The model under review builds one solid part; all positions refer to its coordinate system, in mm. Face numbers are marked on the shaded views. Round coordinates to 2 decimals unless told otherwise and drop trailing zeros. Write each loop counter-clockwise with the first axis right and the second up, starting at its lowest first coordinate (ties: lowest second). Pieces come first, ordered by that corner, then holes. Notation, with made-up numbers: (-26, 19.5) - (11, 19.5) arc R16 cw to (11, 39.5) - close; hole circle Ø6 at (73.5, -32.75). An arc over 180 degrees is marked (long way). Write each question's results on one line, items separated by ' | '.
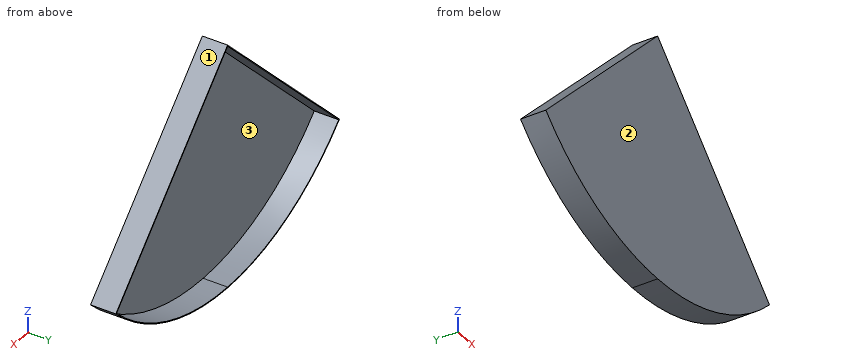
Autodesk Inventor part; units mm, degrees
ref_plane "YZ Plane" through (0, 0, 0) normal (1, 0, 0) x (0, 1, 0)
ref_plane "XZ Plane" through (0, 0, 0) normal (0, 1, 0) x (-1, 0, 0)
ref_plane "XY Plane" through (0, 0, 0) normal (0, 0, 1) x (1, 0, 0)
sketch "草圖1" plane through (0, 0, 0) normal (0, 1, 0) x (-1, 0, 0)
  line L0 (0, 0) -> (-1060.6602, -1060.6602)
  arc A0 (-1060.6602, -1060.6602) -> (0, -1500) centre (0, 0) ccw
  line L1 (0, -1935.3977) -> (0, 330.8159)
  arc A1 (-1067.7254, -1060.6543) -> (0, -1505) centre (0, 0) ccw
  line L2 (-1067.7254, -1060.6543) -> (0, 7.0711)
  line L3 (0, 0) -> (1060.6602, -1060.6602)
  arc A2 (0, -1500) -> (1060.6602, -1060.6602) centre (0, 0) ccw
  arc A3 (0, -1505) -> (1067.7254, -1060.6543) centre (0, 0) ccw
  line L4 (1067.7254, -1060.6543) -> (0, 7.0711)
  dimension "d0" = 45
  dimension "d2" = 1500
  dimension "d3" = 5
  dimension "d5" = 5
extrude "擠出1" add sketch "草圖1" against normal blind 5 contours L1 A0 L0 | L0 A0 L1 A1 L2
extrude "擠出6" add sketch "草圖1" along normal blind 150 contours L0 A0 L1 A1 L2
sketch "草圖29" plane through (0, 0, 0) normal (0, 1, 0) x (1, 0, 0)
  line L0 (0, 0) -> (1060.6602, 1060.6602)
  arc A0 (1060.6602, 1060.6602) -> (0, 1500) centre (0, 0) ccw
  line L1 (0, 1500) -> (0, 0)
mirror "鏡射6" about plane through (0, 0, 0) normal (1, 0, 0) of "擠出1", "擠出6"
properties part number "棒球底座"
Q1. We need section C-C (z = -701.5). State the section outline as (x, y) points, plus the area to 3 significant figures.
Evaluation:
outline: (-708.57, -5) - (708.57, -5) - (708.57, 150) - (701.5, 150) - (701.5, 0) - (-701.5, 0) - (-701.5, 150) - (-708.57, 150) - close | area: 9,210 mm^2
Q2. The part is to be moulded in two halves that separate along X. For the marked faces 1, 2 and 3, say which applies: released by +X, released by -X, zero draft, split by the parting line, or undercut.
Evaluation:
face 1: released by +X | face 2: zero draft | face 3: undercut
Q3. We need section A-A (y = 21.5). State the section outline as (x, z) points, plus the area to 3 significant figures.
Evaluation:
outline: (-1067.73, -1060.65) arc R1505 ccw to (0, -1505) arc R1505 ccw to (1067.73, -1060.65) - (0, 7.07) - close; hole (-1060.66, -1060.66) arc R1500 ccw to (0, -1500) arc R1500 ccw to (1060.66, -1060.66) - (0, 0) - close | area: 26,900 mm^2
Q4. We need section B-B (x = -643). State the section outline as (y, z) points.
Evaluation:
outline: (-5, -1360.73) - (150, -1360.73) - (150, -1355.19) - (0, -1355.19) - (0, -643) - (150, -643) - (150, -635.93) - (-5, -635.93) - close
Q5. Insertion check: P1, Ø5, axis at x = -340, y = 120.5, coming from the +Z side; P2, Ø6, axis at x = -319.5, y = 69, coming from the +Z side; P3, Ø5, axis at y = 77.5, z = -944.5, coming from the +X side. Each pin has a flat end and moves straight along its axis. Give the tip position at first contact, or say it passes through.
Evaluation:
P1: stops at z = -330.43 | P2: stops at z = -309.43 | P3: stops at x = 954.07
Q6. For probe 1 along Y at (x, z) = (678, -973.5); probe 2 along X at (y, z) = (72.5, -538.5); probe 3 along X at (y, z) = (120.5, -798), list the stretches that pass through material, from the lowest coordinate up.
Evaluation:
probe 1: y = -5 to 0 | probe 2: x = -545.57 to -538.5, 538.5 to 545.57 | probe 3: x = -805.07 to -798, 798 to 805.07
